Input: part model. Units: mm. Frame: model coordinates. A direction names the side the tool comes from. Round coordinates to 2 decimals unless told otherwise and drop trailing zeros. Loops run counter-clockwise (first coordinate to the right, second up) from the corner with the lowest first, then second, coordinate; pieces in that order, holes last.
(1) Cut plane D-D, the plane x = -25. Output: boundary loops of the cut face in (y, z).
(2) Cut plane C-C, the plane y = -8. Give the number of separate pieces and of enclosed holes in the cut face, and give its area (3 significant figures).
(3) Cut plane A-A, the plane z = 6.35. Output: boundary loops of the cut face in (x, y) (3 decimals), and give its area (3 significant figures).
(4) Draft query along X for faces 1 (the face through (-35, -9, 17)), 2 (the face through (-24.202, -10.213, 5.397)), 3 (the face through (-30, -9, 0)). Return one class per face: released by +X, released by -X, zero draft, split by the parting line, or undercut.
(5) Access query for faces 4 (the face through (-22.58, -10, 2)), 5 (the face through (-29.207, -8.726, 29.768)), 6 (the face through (-25.755, -8, 7)). Directions: +Z, -Z, +X, -X, +Y, -Y. A direction counts if a zero-diameter tool reaches every point of the face in a straight line with its end or side. Return the directions, or none.
(6) Cut plane B-B, the plane x = -17.5. Output: boundary loops of the cut face in (y, z) (3 decimals), and give its area (3 significant figures).
(7) First-contact query: pin 1 Ø8 at (x, z) = (-7.5, 4) entering from +Y; pin 2 Ø4 at (x, z) = (-6, 20.5) entering from -Y; pin 3 Ø8.5 at (x, z) = (-20, 16.5) entering from +Y. Flat tips, straight axial feed; report the tip coordinate or a pass-through.
(8) Line query: line 1 (Z direction, x = -17.5, y = -10.3); line 2 (X direction, y = -10, z = 30); line 3 (X direction, y = -7, z = 3.5) (3 decimals). Output: solid intervals per line, ascending.
from build123d import *

# Parameters (mm, degrees)
BOSS_EXTRUDE1_DEPTH     = 35
CUT_EXTRUDE4_DEPTH      = 51.280392475
CUT_EXTRUDE4_DEPTH_BACK = 51.280392475
SKETCH6_R               = 1.4732
CUT_EXTRUDE5_DEPTH      = 51.935908437
CUT_EXTRUDE5_DEPTH_BACK = 51.935908437
SKETCH7_R               = 1.4732
CUT_EXTRUDE6_DEPTH      = 52.100782935
SKETCH10_R              = 3.302
CUT_EXTRUDE7_DEPTH      = 40.880823427
SKETCH10_3_R            = 3.302
CUT_EXTRUDE8_DEPTH      = 3.81
SKETCH11_W              = 3.175
SKETCH11_H              = 3.81
CUT_EXTRUDE9_DEPTH      = 50.649791979


with BuildPart() as part:
    # Sketch1 → Boss-Extrude1 (new body)
    with BuildSketch(Plane.XY):
        with BuildLine():
            Line((-35, 0), (-35, -12.7))
            ThreePointArc((-35, -12.7), (-17.5, -11.353892856), (0, -12.7))
            Line((0, -12.7), (0, 0))
            Line((0, 0), (-35, 0))
        make_face()
    extrude(amount=BOSS_EXTRUDE1_DEPTH)

    # Sketch6 → Cut-Extrude4 (cut, two sides: drawn at the far end of the back side and taken through both)
    with BuildSketch(Plane(origin=(-1.080773401, -12.353296496, 0), x_dir=(0.9961946980917455, -0.08715574274765824, 0), z_dir=(-0.08715574274765824, -0.9961946980917455, 0)).offset(-CUT_EXTRUDE4_DEPTH_BACK)):
        with Locations((-6.482080767, 29.70276)):
            Circle(SKETCH6_R)
    extrude(amount=CUT_EXTRUDE4_DEPTH + CUT_EXTRUDE4_DEPTH_BACK, mode=Mode.SUBTRACT)

    # Sketch7 → Cut-Extrude5 (cut, two sides: drawn at the far end of the back side and taken through both)
    with BuildSketch(Plane(origin=(0.814909078, -9.314453387, 0), x_dir=(0.9961946980917455, 0.08715574274765851, 0), z_dir=(0.08715574274765851, -0.9961946980917455, 0)).offset(-CUT_EXTRUDE5_DEPTH_BACK)):
        with Locations((-28.384733667, 29.70276)):
            Circle(SKETCH7_R)
    extrude(amount=CUT_EXTRUDE5_DEPTH + CUT_EXTRUDE5_DEPTH_BACK, mode=Mode.SUBTRACT)

    # Sketch8 → Cut-Extrude6 (cut, through all)
    with BuildSketch(Plane(origin=(0, 0, 0), x_dir=(-1, 0, 0), z_dir=(0, 0, -1))):
        with BuildLine():
            ThreePointArc((0, -6.35), (17.5, -5.003892856), (35, -6.35))
            Line((35, -6.35), (35, 0))
            Line((35, 0), (0, 0))
            Line((0, 0), (0, -6.35))
        make_face()
    extrude(amount=-CUT_EXTRUDE6_DEPTH, mode=Mode.SUBTRACT)

    # Sketch10 → Cut-Extrude7 (cut, through all)
    with BuildSketch(Plane(origin=(-17.5, -5.003892856, 0), x_dir=(-1, 0, 0), z_dir=(0, 1, 0))):
        with Locations((0, 19.05)):
            Circle(SKETCH10_R)
        with Locations((0, 6.35)):
            Circle(SKETCH10_R)
    extrude(amount=-CUT_EXTRUDE7_DEPTH, mode=Mode.SUBTRACT)

    # Sketch10_3 → Cut-Extrude8 (cut)
    # profile 1 of 7: a face of its own
    with BuildSketch(Plane(origin=(-17.5, -5.003892856, 0), x_dir=(-1, 0, 0), z_dir=(0, 1, 0))):
        with BuildLine():
            Line((-8.255, 19.05), (-8.255, 6.35))
            ThreePointArc((-8.255, 6.35), (0, -1.905), (8.255, 6.35))
            Line((8.255, 6.35), (8.255, 19.05))
            ThreePointArc((8.255, 19.05), (0, 27.305), (-8.255, 19.05))
        make_face()
        with BuildLine():
            ThreePointArc((-6.985, 6.35), (0, -0.635), (6.985, 6.35))
            Line((6.985, 6.35), (6.985, 19.05))
            ThreePointArc((6.985, 19.05), (0, 26.035), (-6.985, 19.05))
            Line((-6.985, 19.05), (-6.985, 6.35))
        make_face(mode=Mode.SUBTRACT)
    # profile 2 of 7: a face of its own
    with BuildSketch(Plane(origin=(-17.5, -5.003892856, 0), x_dir=(-1, 0, 0), z_dir=(0, 1, 0))):
        with BuildLine():
            Line((-6.985, 19.05), (-6.985, 6.35))
            ThreePointArc((-6.985, 6.35), (0, -0.635), (6.985, 6.35))
            Line((6.985, 6.35), (6.985, 19.05))
            ThreePointArc((6.985, 19.05), (0, 26.035), (-6.985, 19.05))
        make_face()
        with Locations((0, 19.05)):
            Circle(SKETCH10_3_R, mode=Mode.SUBTRACT)
        with Locations((0, 6.35)):
            Circle(SKETCH10_3_R, mode=Mode.SUBTRACT)
    # profile 3 of 7: a face of its own
    with BuildSketch(Plane(origin=(-17.5, -5.003892856, 0), x_dir=(-1, 0, 0), z_dir=(0, 1, 0))):
        with BuildLine():
            Line((-8.255, 0), (-5.274706153, 0))
            ThreePointArc((-5.274706153, 0), (-7.472875092, 2.842698637), (-8.255, 6.35))
            Line((-8.255, 6.35), (-8.255, 0))
        make_face()
    # profile 4 of 7: a face of its own
    with BuildSketch(Plane(origin=(-17.5, -5.003892856, 0), x_dir=(-1, 0, 0), z_dir=(0, 1, 0))):
        with BuildLine():
            ThreePointArc((5.274706153, 0), (0, -1.905), (-5.274706153, 0))
            Line((-5.274706153, 0), (-8.255, 0))
            Line((-8.255, 0), (-8.255, -2.465000046))
            Line((-8.255, -2.465000046), (8.255, -2.465000046))
            Line((8.255, -2.465000046), (8.255, 0))
            Line((8.255, 0), (5.274706153, 0))
        make_face()
    # profile 5 of 7: a face of its own
    with BuildSketch(Plane(origin=(-17.5, -5.003892856, 0), x_dir=(-1, 0, 0), z_dir=(0, 1, 0))):
        with BuildLine():
            ThreePointArc((8.255, 6.35), (7.472875092, 2.842698637), (5.274706153, 0))
            Line((5.274706153, 0), (8.255, 0))
            Line((8.255, 0), (8.255, 6.35))
        make_face()
    # profile 6 of 7: a face of its own
    with BuildSketch(Plane(origin=(-17.5, -5.003892856, 0), x_dir=(-1, 0, 0), z_dir=(0, 1, 0))):
        with BuildLine():
            ThreePointArc((2.909935566, 0), (0, -0.635), (-2.909935566, 0))
            Line((-2.909935566, 0), (-5.274706153, 0))
            ThreePointArc((-5.274706153, 0), (0, -1.905), (5.274706153, 0))
            Line((5.274706153, 0), (2.909935566, 0))
        make_face()
    # profile 7 of 7: a face of its own
    with BuildSketch(Plane(origin=(-17.5, -5.003892856, 0), x_dir=(-1, 0, 0), z_dir=(0, 1, 0))):
        with BuildLine():
            Line((2.909935566, 0), (-2.909935566, 0))
            ThreePointArc((-2.909935566, 0), (0, -0.635), (2.909935566, 0))
        make_face()
    extrude(amount=-CUT_EXTRUDE8_DEPTH, mode=Mode.SUBTRACT)

    # Sketch11 → Cut-Extrude9 (cut, through all)
    with BuildSketch(Plane(origin=(0, -8.813892856, 0), x_dir=(1, 0, 0), z_dir=(0, 1, 0))):
        with Locations((-24.1675, -1.905)):
            Rectangle(SKETCH11_W, SKETCH11_H)
        with BuildLine():
            ThreePointArc((-25.755, -3.81), (-24.1675, -5.3975), (-22.58, -3.81))
            Line((-22.58, -3.81), (-25.755, -3.81))
        make_face()
    extrude(amount=-CUT_EXTRUDE9_DEPTH, mode=Mode.SUBTRACT)


solid = part.part
Reported:
1. outline: (-11.6, 5.16) - (-8.81, 5.16) - (-8.81, 22.5) - (-5.25, 22.5) - (-5.25, 35) - (-11.6, 35) - close
2. separate pieces: 1
2. enclosed holes: 2
2. area: 790 mm2
3. outline: (-35, -12.7) arc R114.427 cw to (-20.802, -11.402) - (-20.802, -8.814) - (-25.755, -8.814) - (-25.755, -5.302) arc R114.427 ccw to (-35, -6.35) - close; (-14.198, -11.402) arc R114.427 cw to (0, -12.7) - (0, -6.35) arc R114.427 ccw to (-9.245, -5.302) - (-9.245, -8.814) - (-14.198, -8.814) - close
3. area: 144 mm2
4. face 1: released by -X
4. face 2: undercut
4. face 3: zero draft
5. face 4: -Z, +Y, -Y
5. face 5: none
5. face 6: -Z, +Y
6. outline: (-11.354, 0) - (-8.814, 0) - (-8.814, 3.048) - (-11.354, 3.048) - close; (-11.354, 9.652) - (-8.814, 9.652) - (-8.814, 15.748) - (-11.354, 15.748) - close; (-11.354, 22.352) - (-8.814, 22.352) - (-8.814, 27.305) - (-5.004, 27.305) - (-5.004, 35) - (-11.354, 35) - close
6. area: 84.7 mm2
7. pin 1: stops at y = -5.3
7. pin 2: stops at y = -12.15
7. pin 3: stops at y = -8.81
8. line 1: z = 0 to 3.05, 9.65 to 15.75, 22.35 to 35
8. line 2: x = -35 to -29.07, -26.17 to -8.83, -5.93 to 0
8. line 3: x = -35 to -25.755, -9.245 to 0
